```python
from build123d import *

# Parameters (mm, degrees)
SKETCH1_W               = 30
SKETCH1_H               = 30
SKETCH1_W_2             = 7
SKETCH1_H_2             = 26
BOSS_EXTRUDE3_DEPTH     = 90
SKETCH6_R               = 12.7
CUT_EXTRUDE5_DEPTH      = 23
SKETCH8_R               = 3.6
SKETCH8_R_2             = 1.7
CUT_EXTRUDE6_DEPTH      = 17
SKETCH9_W               = 12
SKETCH9_H               = 26
CUT_EXTRUDE7_DEPTH      = 59
M3_CLEARANCE_HOLE1_D    = 3.4
CUT_EXTRUDE8_DEPTH      = 28
CUT_EXTRUDE8_DEPTH_BACK = 26


with BuildPart() as part:
    # Sketch1 → Boss-Extrude3 (new body)
    with BuildSketch(Plane(origin=(0, 0, 0), x_dir=(0, 0, -1), z_dir=(1, 0, 0))):
        Rectangle(SKETCH1_W, SKETCH1_H)
        with Locations((-9.5, 0)):
            Rectangle(SKETCH1_W_2, SKETCH1_H_2, mode=Mode.SUBTRACT)
        with Locations((9.5, 0)):
            Rectangle(SKETCH1_W_2, SKETCH1_H_2, mode=Mode.SUBTRACT)
    extrude(amount=BOSS_EXTRUDE3_DEPTH)

    # Sketch6 → Cut-Extrude5 (cut)
    with BuildSketch(Plane(origin=(0, 0, -15), x_dir=(-1, 0, 0), z_dir=(0, 0, -1))):
        with Locations((-75, 0)):
            Circle(SKETCH6_R)
    extrude(amount=-CUT_EXTRUDE5_DEPTH, mode=Mode.SUBTRACT)

    # Sketch8 → Cut-Extrude6 (cut)
    with BuildSketch(Plane.XY.offset(15)):
        with Locations((75, 0)):
            Circle(SKETCH8_R)
        with Locations((75, 8.5)):
            Circle(SKETCH8_R_2)
        with Locations((75, -8.5)):
            Circle(SKETCH8_R_2)
    extrude(amount=-CUT_EXTRUDE6_DEPTH, mode=Mode.SUBTRACT)

    # Sketch9 → Cut-Extrude7 (cut)
    with BuildSketch(Plane.ZY):
        Rectangle(SKETCH9_W, SKETCH9_H)
    extrude(amount=-CUT_EXTRUDE7_DEPTH, mode=Mode.SUBTRACT)

    # M3 Clearance Hole1 (through all)
    with Locations(Plane.XY.offset(15)):
        with Locations((25, 10), (5, -10), (25, -10), (5, 10)):
            Hole(M3_CLEARANCE_HOLE1_D / 2)

    # Sketch13 → Cut-Extrude8 (cut, two sides)
    with BuildSketch(Plane.XY) as cut_extrude8_sk:
        Polygon((0, -15), (0, 5.364675298), (20.364675298, -15), align=None)
    extrude(amount=CUT_EXTRUDE8_DEPTH, mode=Mode.SUBTRACT)
    extrude(cut_extrude8_sk.sketch, amount=-CUT_EXTRUDE8_DEPTH_BACK, mode=Mode.SUBTRACT)


solid = part.part
```
Here's how the part is built. I have some questions about the finished solid (model axes, mm). A direction names the side the tool comes from. Round coordinates to 2 decimals unless told otherwise and drop trailing zeros. Order: outer loops, then holes, each group sorted by start corner. A loop starts at its lowest first (then second) coordinate and runs counter-clockwise, first axis right, second up. Notation, with made-up numbers: M 53,43.5 L 76,43.5 A31 ccw 76,79.5 Z; hole C 14.5,74.5 d11. An arc over 180 degrees is marked long. One line per question, with ' | ' between items.
1) I need wall thicknesses on line 1 along Z through (x, y) = (62, -3.25); line 2 along Y through (x, z) = (75, 13.7); line 3 along Y through (x, z) = (74, 8.5). Which ranges of each line are inside material? Lowest first, please.
Working result:
line 1: -15 to -13, -6 to 6, 13 to 15 | line 2: -15 to -10.2, -6.8 to -3.6, 3.6 to 6.8, 10.2 to 15 | line 3: -15 to -13, 13 to 15
2) I want a section at C-C, the plane z = -3. Write out the boundary of the cut face in (x, y).
Working result:
outline: M 0,13 L 59,13 L 59,-13 L 18.36,-13 L 20.36,-15 L 90,-15 L 90,15 L 0,15 Z; hole C 75,0 d25.4
3) I want a section at D-D, the plane y = -1. Write out the boundary of the cut face in (x, z).
Working result:
outline: M 6.36,-15 L 62.34,-15 L 62.34,-13 L 6.36,-13 Z; M 6.36,13 L 71.54,13 L 71.54,15 L 6.36,15 Z; M 59,-6 L 62.34,-6 L 62.34,6 L 59,6 Z; M 78.46,13 L 90,13 L 90,15 L 78.46,15 Z; M 87.66,-15 L 90,-15 L 90,-13 L 87.66,-13 Z; M 87.66,-6 L 90,-6 L 90,6 L 87.66,6 Z
4) For faces 1 (the face through (19.186, -13.821, -0.07)), 2 (the face through (59, 0, 0)), 3 (the face through (87.688, 0.558, -0.084)), 4 (the face through (73.3, 8.57, 14.01)), 5 (the face through (67, 11, 6)), which set-ups out of +Z, -Z, +X, -X, +Y, -Y let a thin tool reach every point of the face, with its end or its side?
Working result:
face 1: +Z, -Z, -X, -Y | face 2: -X | face 3: -Z | face 4: +Z, -Z | face 5: +X, -X
5) For pin 1 Ø4.5 at (x, y) = (75, 8.5) entering from -Z; pin 2 Ø12 at (y, z) = (-5.5, 11.5) entering from -X; pin 3 Ø2 at (y, z) = (-2.5, 1.5) entering from -X; pin 4 Ø5.5 at (x, y) = (75, -8.5) entering from +Z, each with a flat end and sliding along its axis, tell me the tip position at first contact or that it passes through.
Working result:
pin 1: z = 13 | pin 2: x = 5.06 | pin 3: x = 59 | pin 4: z = 15
6) I want a section at B-B, the plane z = 11.5. Write out the boundary of the cut face in (x, y).
Working result:
outline: M 0,13 L 90,13 L 90,15 L 0,15 Z; M 18.36,-13 L 20.36,-15 L 90,-15 L 90,-13 Z
7) I want a section at A-A, the plane x = 75. State how many separate pieces and enclosed holes the cut face has, then the cut area to 3 significant figures.
Working result:
separate pieces: 4 | enclosed holes: 0 | area: 152 mm²
8) If we mould it in two halves opening along Y, with no side actions, what happens to faces 6 (the face through (44, 0, 13)), 7 (the face through (0, 13.5, 0.2)), 8 (the face through (87.688, 0.558, -14.014)), 9 (the face through (44, 15, 0))? For each: +Y half, -Y half, draft (parallel to the pull), parting line (faces both ways), or undercut.
Working result:
face 6: undercut | face 7: draft | face 8: undercut | face 9: +Y half
